Could you check a few things on this drawing? It's one solid part, dimensions in mm from its lowest x, y, z. Coordinates: 2 decimals unless noted, no trailing zeros. Loops run counter-clockwise (first coordinate to the right, second up) from the corner with the lowest first, then second, coordinate; pieces in that order, holes last. Notation, with made-up numbers: (59, 24.5) -> (102, 24.5) arc R22 ccw to (102, 31.5) -> close; hole circle Ø6 at (-29.5, 48). An arc over 180 degrees is marked (long way). One line per question, with ' | ' between items. Start each with the question number.
(1) Suppose I cut it at A-A (x = 7). Please give me the cut outline in (y, z).
(2) If I drill on line 1 along Z through (x, y) = (63, 0.75); line 2 along X through (y, z) = (0.7, 25); line 3 along X through (y, z) = (0.7, 22.5) (1 decimal), over which ranges is the centre line in solid material (lowest first)?
(3) I'm going to push a flat-ended pin straight in: pin 1 Ø2 at (x, z) = (63, 23.91) entering from -Y. Where does the tip first touch, or does it pass through?
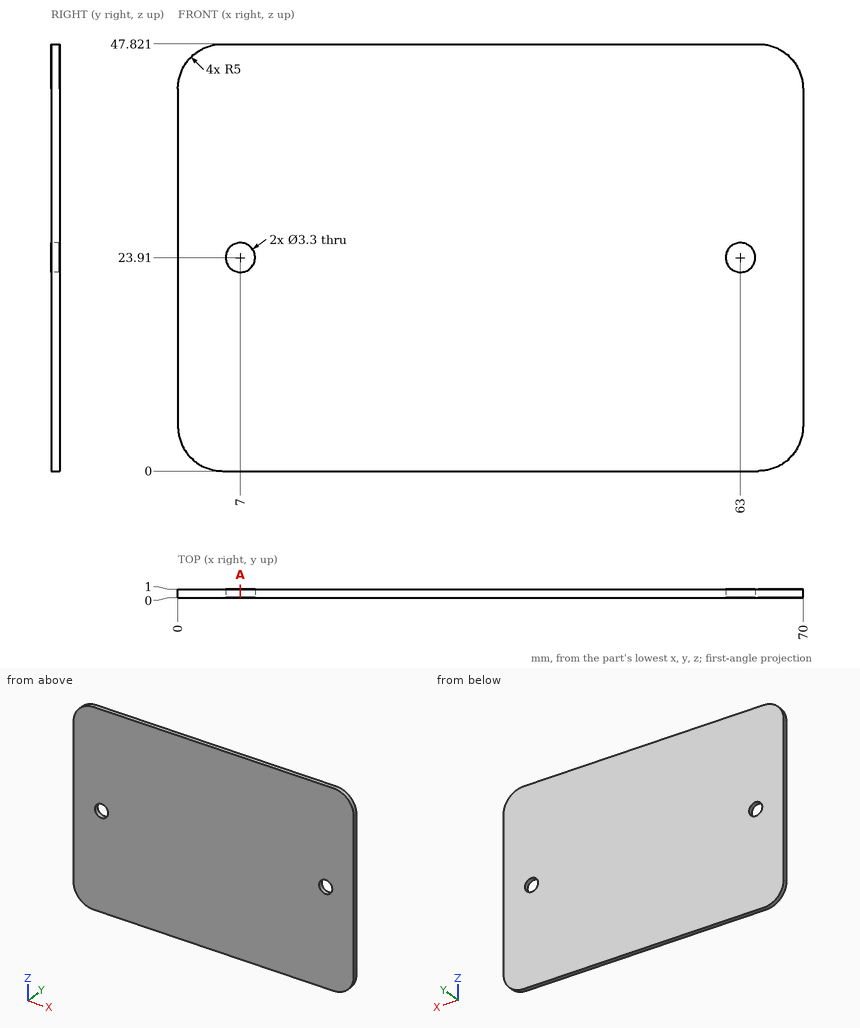
Checks:
1) outline: (0, 0) -> (1, 0) -> (1, 22.26) -> (0, 22.26) -> close; (0, 25.56) -> (1, 25.56) -> (1, 47.82) -> (0, 47.82) -> close
2) line 1: z = 0 to 22.26, 25.56 to 47.82 | line 2: x = 0 to 5.76, 8.24 to 61.76, 64.24 to 70 | line 3: x = 0 to 6.1, 7.9 to 62.1, 63.9 to 70
3) pin 1: passes through
